Geometry check sheet. Reference: drawing and pictorial views, mm from the part's lowest x, y, z. Round coordinates to 2 decimals unless told otherwise and drop trailing zeros. Order: outer loops, then holes, each group sorted by start corner. A loop starts at its lowest first (then second) coordinate and runs counter-clockwise, first axis right, second up.
(1) Cross-section at A-A on x = 17.5. Enter the section's corners in (y, z).
(2) Cross-section at C-C on z = 12. Enter the section's corners in (x, y).
(3) Thickness scan on L1, parallel to Y at x = 17.5, z = 13.25; L2, parallel to Z at x = 28, y = 24.5; L3, parallel to Y at x = 31, z = 13.25. Record the ranges inside material, lowest first.
(4) Draft check along Y on the marked faces 1, 2 and 3. Enter one of: pulls with the +Y half, pulls with the -Y half, needs draft (parallel to the pull), parting line crosses it, or undercut.
(5) Gauge pin test, flat ends, axial feed: P1, Ø1, axis at y = 12, z = 14.5, coming from the +X side; P2, Ø1, axis at x = 7, z = 17, coming from the -Y side; P3, Ø4, axis at x = 9, z = 3, coming from the -Y side. Record the tip position at first contact, or that the pin passes through.
(6) Cross-section at D-D on z = 17. Enter the section's corners in (x, y).
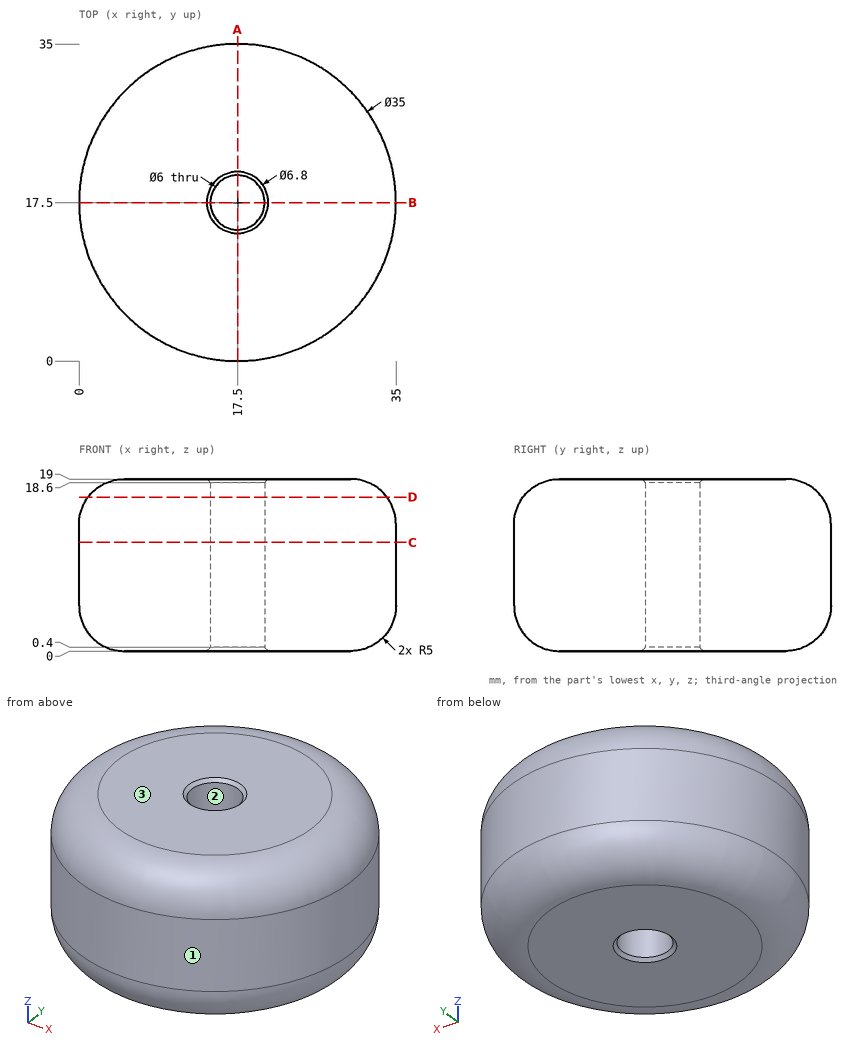
Found:
1. outline: (0, 5) arc R5 ccw to (5, 0) - (14.1, 0) - (14.5, 0.4) - (14.5, 18.6) - (14.1, 19) - (5, 19) arc R5 ccw to (0, 14) - close; (20.5, 0.4) - (20.9, 0) - (30, 0) arc R5 ccw to (35, 5) - (35, 14) arc R5 ccw to (30, 19) - (20.9, 19) - (20.5, 18.6) - close
2. outline: circle Ø35 at (17.5, 17.5); hole circle Ø6 at (17.5, 17.5)
3. L1: y = 0 to 14.5, 20.5 to 35
3. L2: z = 0 to 19
3. L3: y = 6.36 to 28.64
4. face 1: parting line crosses it
4. face 2: undercut
4. face 3: needs draft
5. P1: stops at x = 34.25
5. P2: stops at y = 4.18
5. P3: stops at y = 1.47
6. outline: circle Ø33 at (17.5, 17.5); hole circle Ø6 at (17.5, 17.5)
